Check sheet for the modelled part. Datum: model origin and axes. Units: mm. Round coordinates to 2 decimals unless told otherwise and drop trailing zeros. Order: outer loops, then holes, each group sorted by start corner. A loop starts at its lowest first (then second) coordinate and runs counter-clockwise, first axis right, second up.
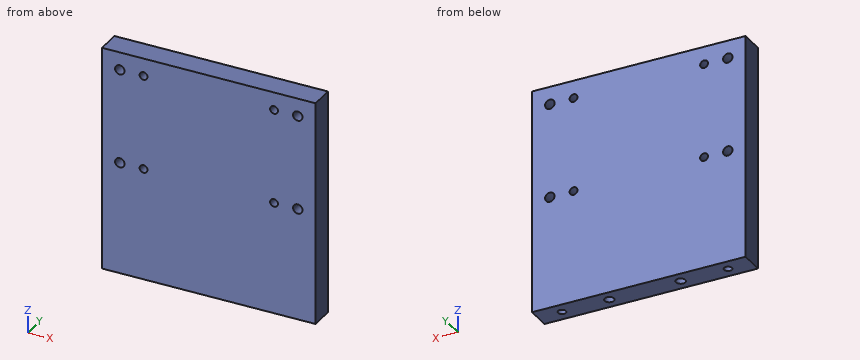
```python
from build123d import *

# Parameters (mm, degrees)
F0_W     = 90
F0_H     = 10
F1_DEPTH = 95
F2_R     = 2
F3_DEPTH = 10
F4_D     = 3.3
F4_DEPTH = 13
F4_TIP   = 0.9914200214
F5_R     = 2
F6_DEPTH = 10.001
F7_D     = 3.3


with BuildPart() as f1:
    # F0 (on Top) → F1 (new body)
    with BuildSketch(Plane.XY):
        Rectangle(F0_W, F0_H)
    extrude(amount=F1_DEPTH)

    # F2 (on face) → F3 (cut)
    with BuildSketch(Plane(origin=(0, 0, 0), x_dir=(1, 0, 0), z_dir=(0, 0, -1))):
        with Locations((-15, 0)):
            Circle(F2_R)
        with Locations((15, 0)):
            Circle(F2_R)
    extrude(amount=-F3_DEPTH, mode=Mode.SUBTRACT)

    # F4
    with Locations(Plane(origin=(0, 0, 0), x_dir=(1, 0, 0), z_dir=(0, 0, -1))):
        with Locations((-35, 0), (35, 0)):
            Hole(F4_D / 2, depth=F4_DEPTH)
            with Locations((0, 0, -(F4_DEPTH + F4_TIP / 2))):  # 118° drill point
                Cone(0, F4_D / 2, F4_TIP, mode=Mode.SUBTRACT)

    # F5 (on face) → F6 (cut, through all)
    with BuildSketch(Plane.XZ.offset(5)):
        with Locations((-37.5, 47.5)):
            Circle(F5_R)
        with Locations((-37.5, 87.5)):
            Circle(F5_R)
        with Locations((37.5, 87.5)):
            Circle(F5_R)
        with Locations((37.5, 47.5)):
            Circle(F5_R)
    extrude(amount=-F6_DEPTH, mode=Mode.SUBTRACT)

    # F7 (through all)
    with Locations(Plane.XZ.offset(5)):
        with Locations((-27.5, 47.5), (-27.5, 87.5), (27.5, 87.5), (27.5, 47.5)):
            Hole(F7_D / 2)


solid = f1.part
```
Item 1: Sectioned sample at A-A (z = 47.5). Record the cut outline in (x, y), and give its area (3 significant figures).
Answer:
outline: (-45, -5) - (-39.5, -5) - (-39.5, 5) - (-45, 5) - close; (-35.5, -5) - (-29.15, -5) - (-29.15, 5) - (-35.5, 5) - close; (-25.85, -5) - (25.85, -5) - (25.85, 5) - (-25.85, 5) - close; (29.15, -5) - (35.5, -5) - (35.5, 5) - (29.15, 5) - close; (39.5, -5) - (45, -5) - (45, 5) - (39.5, 5) - close
area: 754 mm2
Item 2: Sectioned sample at C-C (x = 15). Record the cut outline in (y, z).
Answer:
outline: (-5, 0) - (-2, 0) - (-2, 10) - (2, 10) - (2, 0) - (5, 0) - (5, 95) - (-5, 95) - close
Item 3: Scan lines: line 1 along Z through (x, y) = (-27.5, -2.75); line 2 along Y through (x, z) = (-35, 9.5); line 3 along Y through (x, z) = (-15, 6.5). Record each from-to range of solid material in increasing order.
Answer:
line 1: z = 0 to 45.85, 49.15 to 85.85, 89.15 to 95
line 2: y = -5 to -1.65, 1.65 to 5
line 3: y = -5 to -2, 2 to 5
Item 4: Sectioned sample at B-B (x = 27.5). Record the cut outline in (y, z), and give its area (3 significant figures).
Answer:
outline: (-5, 0) - (5, 0) - (5, 45.85) - (-5, 45.85) - close; (-5, 49.15) - (5, 49.15) - (5, 85.85) - (-5, 85.85) - close; (-5, 89.15) - (5, 89.15) - (5, 95) - (-5, 95) - close
area: 884 mm2
Item 5: Go/stop test with flat-tipped pins: P1, Ø3.5, axis at x = -37.5, z = 47.5, coming from the -Y side; P2, Ø3, axis at x = 15, y = 0, coming from the -Z side. Record where each tip stops, or that it passes through.
Answer:
P1: passes through
P2: stops at z = 10
